Design review of the part shown in the three views and the two pictorial views. Dimensions are in mm from the part's minimum x, y and z. Give positions to 0.01 mm unless a question says otherwise; leave off trailing zeros. Loops run counter-clockwise (first coordinate to the right, second up) from the corner with the lowest first, then second, coordinate; pieces in that order, holes last. Notation, with made-up numbers: (21, 85) -> (32, 85) arc R35 cw to (32, 123) -> close; hole circle Ø4 at (63.5, 57). An arc over 180 degrees is marked (long way). Use CSV: the item, a comma, the result in double quotes. Start each with the question number.
Item 1: We need section C-C (y = 5). State the section outline as (x, z) points, plus the area to 3 significant figures.
Item 2: Wall thickness on line 1 along X through (y, z) = (4.75, 15); line 2 along X through (y, z) = (0.8, 45); line 3 along Z through (x, y) = (68, 7.75): over which ranges is each line inside the solid? List them lowest first. Write a range as from..to.
Item 3: We need section A-A (x = 50). State the section outline as (y, z) points, plus the area to 3 significant figures.
Item 4: Clearance check with flat-ended pins moving along their axes: pin 1 (2 mm diameter, centred on x = 32, z = 45, fed in from +Y); pin 2 (2 mm diameter, centred on x = 69, z = 45.5, fed in from -Y). State where each tip first meets the part, or that it passes through.
Item 5: The part is to be moulded in two halves that separate along Z. For the marked faces 1, 2 and 3, say which applies: +Z half, -Z half, draft (parallel to the pull), parting line (faces both ways), or undercut.
Item 6: We need section B-B (z = 15). State the section outline as (x, y) points.
Item 7: We need section D-D (z = 45). State the section outline as (x, y) points.
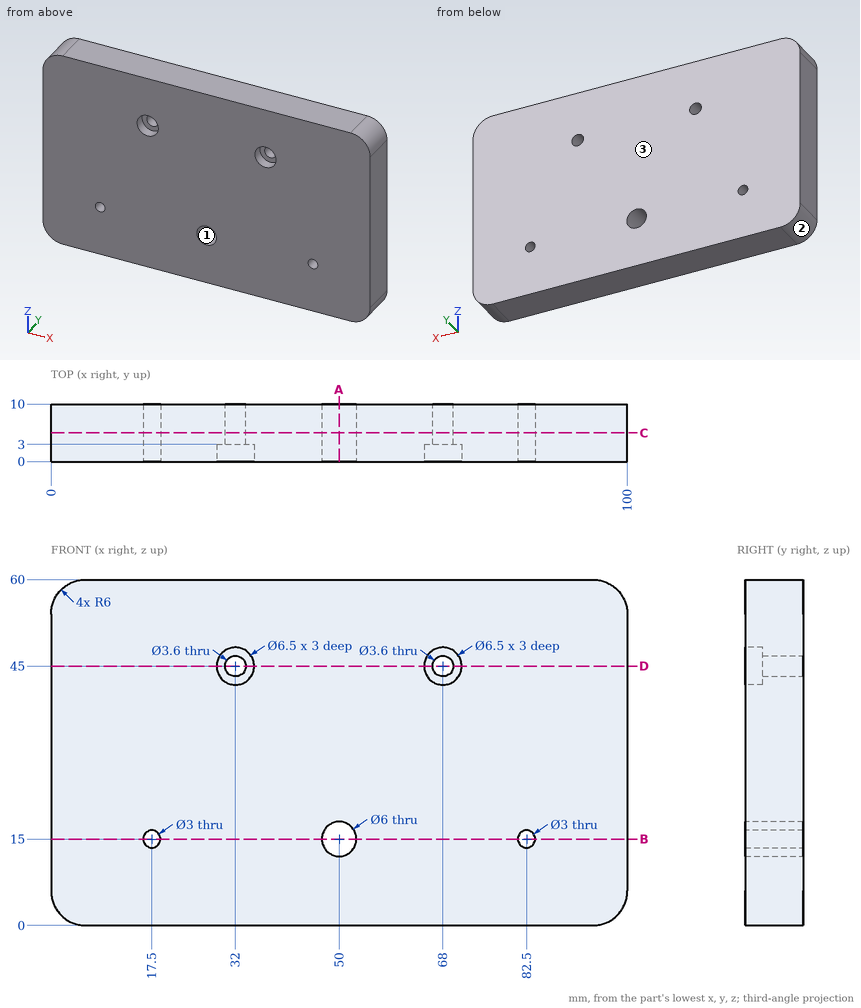
Results found:
1,outline,"(0, 6) arc R6 ccw to (6, 0) -> (94, 0) arc R6 ccw to (100, 6) -> (100, 54) arc R6 ccw to (94, 60) -> (6, 60) arc R6 ccw to (0, 54) -> close; hole circle Ø3 at (17.5, 15); hole circle Ø3.6 at (32, 45); hole circle Ø6 at (50, 15); hole circle Ø3.6 at (68, 45); hole circle Ø3 at (82.5, 15)"
1,area,"5,910 mm²"
2,line 1,"0..16, 19..47, 53..81, 84..100"
2,line 2,"0..28.75, 35.25..64.75, 71.25..100"
2,line 3,"0..43.2, 46.8..60"
3,outline,"(0, 0) -> (10, 0) -> (10, 12) -> (0, 12) -> close; (0, 18) -> (10, 18) -> (10, 60) -> (0, 60) -> close"
3,area,"540 mm²"
4,pin 1,"through"
4,pin 2,"y = 3"
5,face 1,"undercut"
5,face 2,"-Z half"
5,face 3,"draft"
6,outline,"(0, 0) -> (16, 0) -> (16, 10) -> (0, 10) -> close; (19, 0) -> (47, 0) -> (47, 10) -> (19, 10) -> close; (53, 0) -> (81, 0) -> (81, 10) -> (53, 10) -> close; (84, 0) -> (100, 0) -> (100, 10) -> (84, 10) -> close"
7,outline,"(0, 0) -> (28.75, 0) -> (28.75, 3) -> (30.2, 3) -> (30.2, 10) -> (0, 10) -> close; (33.8, 3) -> (35.25, 3) -> (35.25, 0) -> (64.75, 0) -> (64.75, 3) -> (66.2, 3) -> (66.2, 10) -> (33.8, 10) -> close; (69.8, 3) -> (71.25, 3) -> (71.25, 0) -> (100, 0) -> (100, 10) -> (69.8, 10) -> close"
